Solid Edge part; units mm, degrees
sketch "Sketch1" plane through (0, 0, 0) normal (0, 0, 1) x (1, 0, 0)
  line L0 (20, -3) -> (10, -3)
  line L1 (10, -3) -> (10, -4.5)
  line L2 (10, -4.5) -> (5.8772, -4.5)
  arc A0 (5.8772, -4.5) -> (5.0365, -6.0414) centre (5.8772, -5.5) ccw
  line L3 (5.0365, -6.0414) -> (10, -13.75)
  line L4 (10, -13.75) -> (10, -15.25)
  line L5 (8.5, -15.25) -> (10, -15.25)
  line L6 (8.5, -13.75) -> (8.5, -15.25)
  line L7 (0, -13.75) -> (8.5, -13.75)
  line L8 (0, 0) -> (0, -13.75)
  line L9 (0, 0) -> (20, 0)
  line L10 (20, 0) -> (20, -3)
revolve "RevolvedProtrusion1" add sketch "Sketch1" angle 360 about axis through (0, 0, 0) along (1, 0, 0)
sketch "Sketch2" plane through (0, 0, 0) normal (-1, 0, 0) x (0, 0, 1)
  line L0 (-7.433, 1) -> (-19.394, 1)
  line L1 (-19.394, 1) -> (-19.394, 18)
  line L2 (-19.394, 18) -> (-5.9543, 4.5603)
  arc A0 (-5.9543, 4.5603) -> (-7.433, 1) centre (0, 0) ccw
  line L3 (-7.433, -1) -> (-19.394, -1)
  line L4 (-19.394, -1) -> (-19.394, -18)
  line L5 (-19.394, -18) -> (-5.9543, -4.5603)
  arc A1 (-5.9543, -4.5603) -> (-7.433, -1) centre (0, 0) cw
  line L6 (-4.3097, -6.1381) -> (-18, -19.8284)
  line L7 (-18, -19.8284) -> (-1, -19.8284)
  line L8 (-1, -19.8284) -> (-1, -7.433)
  arc A2 (-1, -7.433) -> (-4.3097, -6.1381) centre (0, 0) cw
  line L9 (1, -19.8284) -> (1, -7.433)
  arc A3 (1, -7.433) -> (4.3097, -6.1381) centre (0, 0) ccw
  line L10 (4.3097, -6.1381) -> (18, -19.8284)
  line L11 (18, -19.8284) -> (1, -19.8284)
  line L12 (19.394, -18) -> (5.9543, -4.5603)
  arc A4 (5.9543, -4.5603) -> (7.433, -1) centre (0, 0) ccw
  line L13 (7.433, -1) -> (19.394, -1)
  line L14 (19.394, -1) -> (19.394, -18)
  line L15 (7.433, 1) -> (19.394, 1)
  line L16 (19.394, 1) -> (19.394, 18)
  line L17 (19.394, 18) -> (5.9543, 4.5603)
  arc A5 (5.9543, 4.5603) -> (7.433, 1) centre (0, 0) cw
  line L18 (4.3097, 6.1381) -> (18, 19.8284)
  line L19 (18, 19.8284) -> (1, 19.8284)
  line L20 (1, 19.8284) -> (1, 7.433)
  arc A6 (1, 7.433) -> (4.3097, 6.1381) centre (0, 0) cw
  line L21 (-1, 19.8284) -> (-1, 7.433)
  arc A7 (-1, 7.433) -> (-4.3097, 6.1381) centre (0, 0) ccw
  line L22 (-4.3097, 6.1381) -> (-18, 19.8284)
  line L23 (-18, 19.8284) -> (-1, 19.8284)
extrude "Cutout1" cut sketch "Sketch2" against normal blind 5.9
mirror "Mirror1" about plane through (0, 0, 0) normal (1, 0, 0) of "RevolvedProtrusion1", "Cutout1"
Input: part model. Units: mm. Frame: model coordinates. A direction names the side the tool comes from. Give positions to 0.01 mm unless a question says otherwise; leave off trailing zeros. Write each loop counter-clockwise with the first axis right and the second up, starting at its lowest first coordinate (ties: lowest second). Pieces come first, ordered by that corner, then holes. Notation, with made-up numbers: M -36.5,26 L -18.5,26 A29 cw -18.5,51 Z; hole C 10.5,-16.5 d10. An arc over 180 degrees is marked long. Use one line per item in the form item = value.
1. Cut plane C-C on x = -9. Return loops of the section in (y, z), and give its area (3 significant figures).
Outcome:
outline = C 0,0 d30.5; C 0,0 d9; hole C 0,0 d24.39
area = 327 mm²
2. Cut plane B-B on x = 7.5. Return loops of the section in (y, z).
Outcome:
outline = C 0,0 d27.5; C 0,0 d9; hole C 0,0 d19.73
3. First-contact query: P1, Ø3, axis at x = 3.5, z = 4.5, coming from the -Y side; P2, Ø8.5, axis at y = 11.5, z = 4.5, coming from the -X side; P3, Ø6, axis at y = 5.5, z = -8, coming from the -X side; P4, Ø15, axis at y = 1.5, z = 3.5, coming from the -X side. Flat tips, straight axial feed; report the tip coordinate or a pass-through.
Outcome:
P1 = -7.83
P2 = -10
P3 = -9.33
P4 = -20
4. Reachability of faces 4 (the face through (-5.9, 10, 4)), 5 (the face through (5.9, -10, -4)), 6 (the face through (-0.083, -6.812, 8.206)), 7 (the face through (5.9, 4, -10)) from +Z, -Z, +X, -X, +Y, -Y: full face, straight path, thin tool, end or side. Return the list, or none.
Outcome:
face_4 = +Y
face_5 = -Y
face_6 = +Z
face_7 = -Z
5. Mould query, pull axis X, two halves, no side actions, for faces 1 (the face through (0, -1, 11)), 2 (the face through (-15, 3, 0)), 3 (the face through (-10, -2, -14)). Classes: released by +X, released by -X, zero draft, split by the parting line, or undercut.
Outcome:
face_1 = undercut
face_2 = zero draft
face_3 = released by -X
6. Ray query, L1, parallel to X at y = -12, z = -7.5; L2, parallel to Y at x = 9.5, z = 3; L3, parallel to Y at x = 3, z = 10. Return the intervals inside material, ascending.
Outcome:
L1 = -10 to -8.5, 8.5 to 10
L2 = -14.95 to -12.62, -3.35 to 3.35, 12.62 to 14.95
L3 = -9.44 to -8.61, -1 to 1, 8.61 to 9.44
